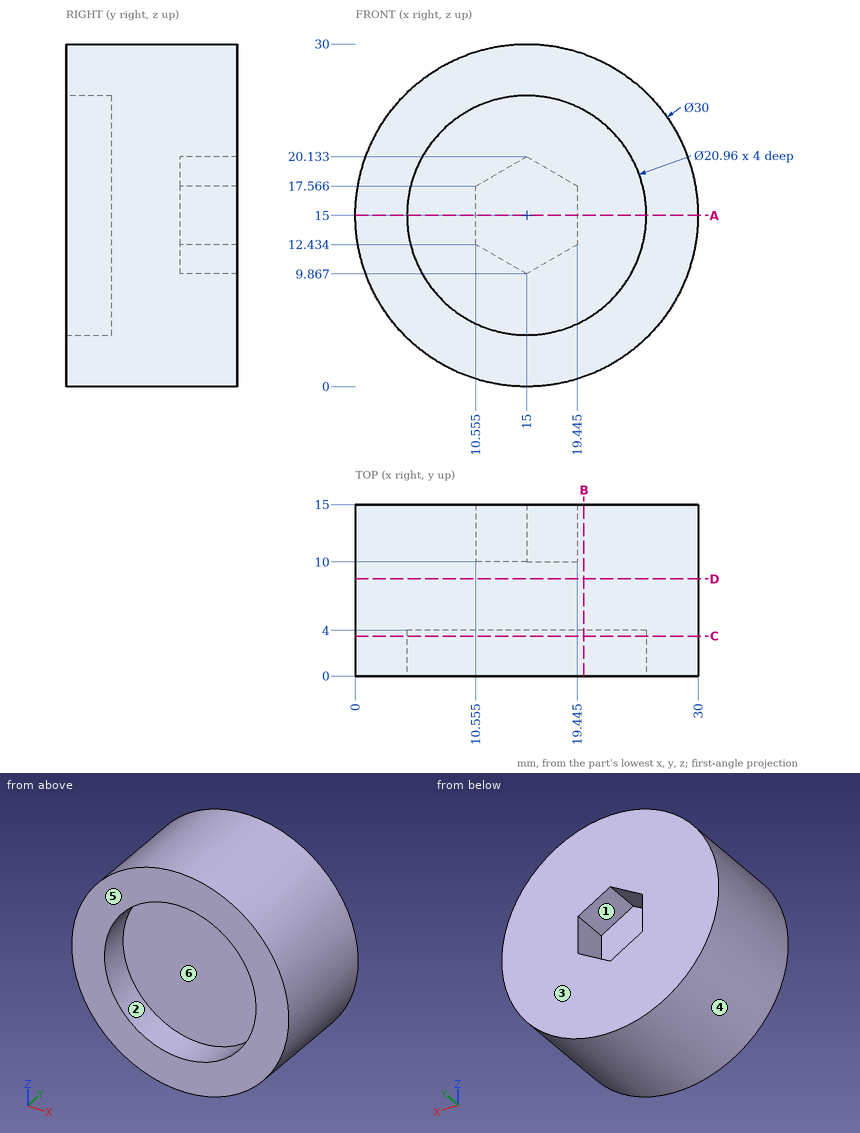
The figure shows three views and two pictorial views of one solid part (mm, origin at its lowest corner). Answer the questions. A direction names the side the tool comes from. Give positions to 0.01 mm unless a question says otherwise; leave off trailing zeros. Write each loop counter-clockwise with the first axis right and the second up, starting at its lowest first coordinate (ties: lowest second). Pieces come first, ordered by that corner, then holes. Notation, with made-up numbers: (48, -28) -> (90, -28) arc R19 ccw to (90, -3) -> close; hole circle Ø11 at (-10, -22.75). An arc over 180 degrees is marked (long way). Write each question's results on one line, items separated by ' | '.
1. Straight lines are drawn through the part: L1, parallel to X at y = 3.2, z = 15; L2, parallel to Y at x = 14.5, z = 21.75; L3, parallel to X at y = 3.5, z = 19.75. For each, find the intervals that lie inside material, in ascending order.
Data:
L1: 0 to 4.52, 25.48 to 30 | L2: 4 to 15 | L3: 0.77 to 5.66, 24.34 to 29.23
2. Each of these flat-tipped pins is pushed along its axis until it touches: pin 1 Ø1 at (x, z) = (14.5, 14) entering from +Y; pin 2 Ø1.5 at (y, z) = (3, 17) entering from +X; pin 3 Ø2 at (y, z) = (10, 20.5) entering from -X. Where does it stop, or does it pass through?
Data:
pin 1: y = 10 | pin 2: x = 29.95 | pin 3: x = 0.69
3. Find section B-B on x = 20. Determine the outline of the cut face in (y, z), and give its area (3 significant figures).
Data:
outline: (0, 0.86) -> (15, 0.86) -> (15, 29.14) -> (0, 29.14) -> (0, 24.21) -> (4, 24.21) -> (4, 5.79) -> (0, 5.79) -> close | area: 351 mm^2
4. Determine the mould class of the marked faces 4, 5 and 6 for opening direction X: +X half, -X half, draft (parallel to the pull), parting line (faces both ways), or undercut.
Data:
face 4: parting line | face 5: draft | face 6: undercut
5. Find section D-D on y = 8.5. Determine the outline of the cut face in (x, z).
Data:
outline: circle Ø30 at (15, 15)
6. A tool of negligible diameter and unlimited length cuts with its end or side. For the marked faces 1, 2 and 3, from which of +Z, -Z, +X, -X, +Y, -Y can it reach the whole face along a straight path? Write none if from no direction.
Data:
face 1: +Y | face 2: -Y | face 3: +Z, -Z, +X, -X, +Y
7. Find section C-C on y = 3.5. Determine the outline of the cut face in (x, z), and give its area (3 significant figures).
Data:
outline: circle Ø30 at (15, 15); hole circle Ø20.96 at (15, 15) | area: 362 mm^2
8. Find section A-A on z = 15. Determine the outline of the cut face in (x, y) (1 decimal), and give its area (3 significant figures).
Data:
outline: (0, 0) -> (4.5, 0) -> (4.5, 4) -> (25.5, 4) -> (25.5, 0) -> (30, 0) -> (30, 15) -> (19.4, 15) -> (19.4, 10) -> (10.6, 10) -> (10.6, 15) -> (0, 15) -> close | area: 322 mm^2
